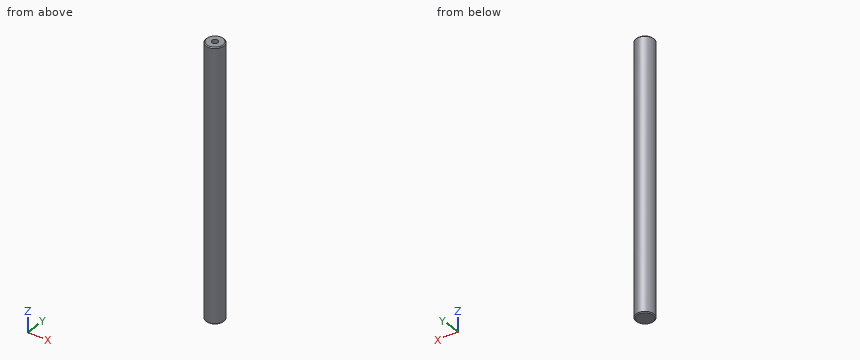
from build123d import *

# Parameters (mm, degrees)
SKETCH1_R             = 10
BOSS_EXTRUDE1_DEPTH   = 150
M8_TAPPED_HOLE1_D     = 6.8
M8_TAPPED_HOLE1_DEPTH = 19.75
M8_TAPPED_HOLE1_TIP   = 2.042926105
CHAMFER1_SIZE         = 1


with BuildPart() as part:
    # Sketch1 → Boss-Extrude1 (new body, symmetric)
    with BuildSketch(Plane.XY):
        Circle(SKETCH1_R)
    extrude(amount=BOSS_EXTRUDE1_DEPTH, both=True)

    # M8 Tapped Hole1
    with Locations(Plane.XY.offset(150)):
        with Locations((0, 0)):
            Hole(M8_TAPPED_HOLE1_D / 2, depth=M8_TAPPED_HOLE1_DEPTH)
            with Locations((0, 0, -(M8_TAPPED_HOLE1_DEPTH + M8_TAPPED_HOLE1_TIP / 2))):  # 118° drill point
                Cone(0, M8_TAPPED_HOLE1_D / 2, M8_TAPPED_HOLE1_TIP, mode=Mode.SUBTRACT)

    # Chamfer1
    chamfer1_edges = [part.edges().sort_by_distance(p)[0] for p in [
        (-10, 0, -150),
        (-10, 0, 150),
    ]]
    chamfer(chamfer1_edges, length=CHAMFER1_SIZE)


solid = part.part
Verification items for the finished model (mm, model axes). Give positions to 0.01 mm unless a question says otherwise; leave off trailing zeros. Loops run counter-clockwise (first coordinate to the right, second up) from the corner with the lowest first, then second, coordinate; pieces in that order, holes last. Notation, with made-up numbers: (32.5, 27) - (43.5, 27) arc R26 cw to (43.5, 42) - close; hole circle Ø5 at (28, 66). An arc over 180 degrees is marked (long way). Write item = value, one per line. Start each with the question number.
Q1. Cross-section at A-A, the plane z = -91.5. Enter the section's corners in (x, y), and give its area (3 significant figures).
Q2. Thickness scan on line 1 (Y direction, x = 0, z = 143); line 2 (X direction, y = 4.25, z = 83); line 3 (Y direction, x = 0, z = -47.5). Record the ranges inside material, lowest first.
Q3. Depth check by flat-ended pin: P1, Ø5, axis at y = 2.5, z = -72, coming from the +X side; P2, Ø2, axis at x = 5.5, z = -84.5, coming from the +Y side; P3, Ø3, axis at x = 8, z = 16.5, coming from the +Y side; P4, Ø1, axis at x = 2.5, z = -44.5, coming from the +Y side. Enter the tip coordinate at first touch or a pass-through.
Answer key:
q1.outline = circle Ø20 at (0, 0)
q1.area = 314 mm^2
q2.line_1 = -10 to -3.4, 3.4 to 10
q2.line_2 = -9.05 to 9.05
q2.line_3 = -10 to 10
q3.P1 = 10
q3.P2 = 8.93
q3.P3 = 7.6
q3.P4 = 9.8
